```python
from build123d import *

# Parameters (mm, degrees)
SKETCH1_W                = 142
SKETCH1_H                = 102
BOSS_EXTRUDE1_DEPTH      = 6
SKETCH2_R                = 38.227
CUT_EXTRUDE1_DEPTH       = 149.182320133
SKETCH4_R                = 2
CUT_EXTRUDE2_DEPTH       = 149.182320133
CIRPATTERN1_COUNT        = 4
SKETCH5_R                = 16.5
CUT_EXTRUDE3_DEPTH       = 149.182320133
FILLET1_R                = 12
F_5_0_5_DIAMETER_HOLE1_D = 4


with BuildPart() as part:
    # Sketch1 → Boss-Extrude1 (new body)
    with BuildSketch(Plane.XY):
        with Locations((68, 0)):
            Rectangle(SKETCH1_W, SKETCH1_H)
    extrude(amount=-BOSS_EXTRUDE1_DEPTH)

    # Sketch2 → Cut-Extrude1 (cut, through all)
    with BuildSketch(Plane.XY):
        with Locations((49, 0)):
            Circle(SKETCH2_R)
    extrude(amount=-CUT_EXTRUDE1_DEPTH, mode=Mode.SUBTRACT)

    # Sketch4 → Cut-Extrude2 (cut, through all)
    with BuildSketch(Plane.XY):
        with Locations((81.880465325, 32.880465325)):
            Circle(SKETCH4_R)
    cut_extrude2 = extrude(amount=-CUT_EXTRUDE2_DEPTH, mode=Mode.SUBTRACT)

    # CirPattern1: Cut-Extrude2 ×4 about axis
    cirpattern1_axis = Axis((49, 0, 0), (0, 0, 1))
    for i in range(1, CIRPATTERN1_COUNT):
        add(cut_extrude2.rotate(cirpattern1_axis, i * 360 / CIRPATTERN1_COUNT), mode=Mode.SUBTRACT)

    # Sketch5 → Cut-Extrude3 (cut, through all)
    with BuildSketch(Plane.XY):
        with Locations((114, 24)):
            Circle(SKETCH5_R)
    extrude(amount=-CUT_EXTRUDE3_DEPTH, mode=Mode.SUBTRACT)

    # Mirror2: part across plane


with BuildPart() as part_1:
    add(part.part)
    add(part.part.mirror(Plane(origin=(0, 0, 0), x_dir=(0, 0, 1), z_dir=(1, 0, 0))))

    # Fillet1
    fillet1_edges = [part_1.edges().sort_by_distance(p)[0] for p in [
        (-139, 51, -3),
        (-139, -51, -3),
        (139, 51, -3),
        (139, -51, -3),
    ]]
    fillet(fillet1_edges, radius=FILLET1_R)

    # Ø5.0 (5) Diameter Hole1 (through all)
    with Locations(Plane.XY):
        with Locations((-130, 42), (130, -42), (-130, -42), (130, 42), (0, 42), (0, -42)):
            Hole(F_5_0_5_DIAMETER_HOLE1_D / 2)


solid = part_1.part
```
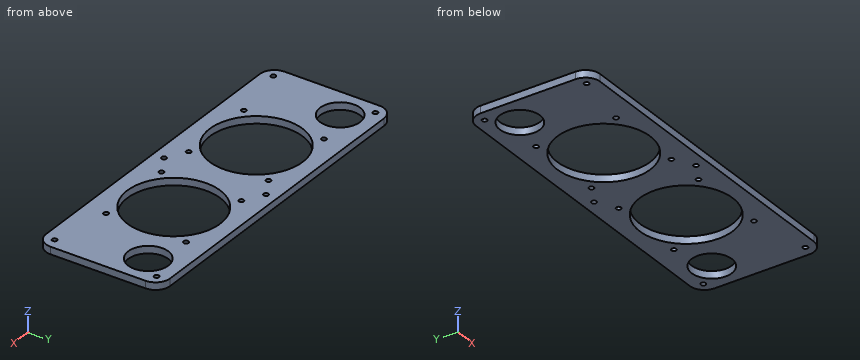
CAD build for the part. Positions are in the model's coordinates, mm. Coordinates: 2 decimals unless noted, no trailing zeros. Write each loop counter-clockwise with the first axis right and the second up, starting at its lowest first coordinate (ties: lowest second). Pieces come first, ordered by that corner, then holes.
(1) Cut at B-B, the plane y = 0. List the corners of the cut face in (x, z), and give its area (3 significant figures).
(2) Cut at A-A, the plane x = -114. List the corners of the cut face in (y, z), and give its area (3 significant figures).
(3) Drill centre lines: probe 1 along Y at (x, z) = (48, -1.9); probe 2 along X at (y, z) = (-8.5, -0.2); probe 3 along X at (y, z) = (22, -2.9). Where is each one in solid material? Low to high.
(4) Cut at C-C, the plane z = -3.75. Count the separate pieces of the cut face and the enclosed holes in it, and give its area (3 significant figures).
(5) Flat gauge pin, fed straight in: pin 1 (3.5 mm diameter, centred on x = 0, y = -42, fed in from +Z). Where does the tip first touch, or does it go through?
(6) Cut at D-D, the plane y = 17.5. List the corners of the cut face in (x, z), and give its area (3 significant figures).
Geometry says:
1. outline: (-139, -6) - (-87.23, -6) - (-87.23, 0) - (-139, 0) - close; (-10.77, -6) - (10.77, -6) - (10.77, 0) - (-10.77, 0) - close; (87.23, -6) - (139, -6) - (139, 0) - (87.23, 0) - close
1. area: 751 mm2
2. outline: (-51, -6) - (7.5, -6) - (7.5, 0) - (-51, 0) - close; (40.5, -6) - (51, -6) - (51, 0) - (40.5, 0) - close
2. area: 414 mm2
3. probe 1: y = -51 to -38.21, 38.21 to 51
3. probe 2: x = -139 to -86.27, -11.73 to 11.73, 86.27 to 139
3. probe 3: x = -139 to -130.38, -97.62 to -80.26, -17.74 to 17.74, 80.26 to 97.62, 130.38 to 139
4. separate pieces: 1
4. enclosed holes: 18
4. area: 17,200 mm2
5. pin 1: passes through
6. outline: (-139, -6) - (-129.17, -6) - (-129.17, 0) - (-139, 0) - close; (-98.83, -6) - (-82.99, -6) - (-82.99, 0) - (-98.83, 0) - close; (-15.01, -6) - (15.01, -6) - (15.01, 0) - (-15.01, 0) - close; (82.99, -6) - (98.83, -6) - (98.83, 0) - (82.99, 0) - close; (129.17, -6) - (139, -6) - (139, 0) - (129.17, 0) - close
6. area: 488 mm2
